```python
from build123d import *

# Parameters (mm, degrees)
SKETCH1_R           = 3.175
BOSS_EXTRUDE1_DEPTH = 6.35


with BuildPart() as part:
    # Sketch1 → Boss-Extrude1 (new body)
    with BuildSketch(Plane.XY):
        with BuildLine():
            Line((63.5, 0), (127, 0))
            ThreePointArc((127, 0), (99.857277989, 28.53470612), (80.244706938, 62.685897436))
            ThreePointArc((80.244706938, 62.685897436), (77.221445945, 72.414145018), (76.2, 82.55))
            Line((76.2, 82.55), (76.2, 101.6))
            Line((76.2, 101.6), (0, 101.6))
            Line((0, 101.6), (0, 63.5))
            ThreePointArc((0, 63.5), (18.598719395, 18.598719395), (63.5, 0))
        make_face()
        with Locations((12.7, 88.9)):
            Circle(SKETCH1_R, mode=Mode.SUBTRACT)
    extrude(amount=BOSS_EXTRUDE1_DEPTH)


solid = part.part
```
Geometry check sheet. Reference: the model listing, model coordinates, mm. A direction names the side the tool comes from. Give positions to 0.01 mm unless a question says otherwise; leave off trailing zeros. Order: outer loops, then holes, each group sorted by start corner. A loop starts at its lowest first (then second) coordinate and runs counter-clockwise, first axis right, second up.
1. Section check C-C, the plane x = 12.7. Enter the section's corners in (y, z) (3 decimals).
2. Thickness scan on L1, parallel to X at y = 82.5, z = 2; L2, parallel to Y at x = 12.7, z = 3.25 (3 decimals); L3, parallel to Y at x = 39.5, z = 4. Record the ranges inside material, lowest first.
3. Section check B-B, the plane z = 1.5. Enter the section's corners in (x, y) (3 decimals), and give its area (3 significant figures).
4. Section check D-D, the plane y = 72. Enter the section's corners in (x, z).
5. Release check for a two-part mould opening along X. For faces 1 (the face through (77.25, 72.27, 3.13)), 2 (the face through (12.01, 85.8, 3.13)), 3 (the face through (48, 52, 6.35)) record: pulls with the +X half, pulls with the -X half, needs draft (parallel to the pull), parting line crosses it, or undercut.
6. Access from +Z, -Z, +X, -X, +Y, -Y to the whole of each face (thin tool, end or side, straight path). Record for faces 4 (the face through (95, 0, 3)), 5 (the face through (76.2, 92, 3)).
7. Section check A-A, the plane y = 88.9. Enter the section's corners in (x, z) (3 decimals).
8. Gauge pin test, flat ends, axial feed: pin 1 Ø6 at (x, y) = (74.5, 81.5) entering from -Z; pin 2 Ø1 at (y, z) = (61.5, 0.5) entering from +X. Record the tip position at first contact, or that the pin passes through.
Values follow:
1. outline: (25.4, 0) - (85.725, 0) - (85.725, 6.35) - (25.4, 6.35) - close; (92.075, 0) - (101.6, 0) - (101.6, 6.35) - (92.075, 6.35) - close
2. L1: x = 0 to 76.2
2. L2: y = 25.4 to 85.725, 92.075 to 101.6
2. L3: y = 4.71 to 101.6
3. outline: (0, 63.5) arc R63.5 ccw to (63.5, 0) - (127, 0) arc R165.1 cw to (80.245, 62.686) arc R50.8 cw to (76.2, 82.55) - (76.2, 101.6) - (0, 101.6) - close; hole circle Ø6.35 at (12.7, 88.9)
3. area: 8,340 mm2
4. outline: (0, 0) - (77.31, 0) - (77.31, 6.35) - (0, 6.35) - close
5. face 1: pulls with the +X half
5. face 2: undercut
5. face 3: needs draft
6. face 4: +Z, -Z, +X, -X, -Y
6. face 5: +Z, -Z, +X, +Y
7. outline: (0, 0) - (9.525, 0) - (9.525, 6.35) - (0, 6.35) - close; (15.875, 0) - (76.2, 0) - (76.2, 6.35) - (15.875, 6.35) - close
8. pin 1: stops at z = 0
8. pin 2: stops at x = 80.97
